Can you work these out from the drawing? Everything is in mm from the part's minimum corner. Coordinates: 2 decimals unless noted, no trailing zeros. Loops run counter-clockwise (first coordinate to the right, second up) from the corner with the lowest first, then second, coordinate; pieces in that order, holes last. Notation, with made-up numbers: M -28.75,-32.75 L 24.25,-32.75 A17 ccw 24.25,-15.75 Z; hole C -35.5,49.5 d11. An arc over 180 degrees is marked long. Use CSV: the item, a comma, the result in double quotes. Start each with the question number.
Q1. Please list where these lines run through material, in increasing order: probe 1 along X at (y, z) = (12.5, 107.95); probe 2 along Z at (x, y) = (58, 2); probe 3 along Z at (x, y) = (20.5, 3.75). Write a range as [from, to].
Q2. If we section it at A-A (z = 19.05): Please give me the cut outline in (x, y).
Q3. If we section it at D-D (x = 57.15): Please give me the cut outline in (y, z).
Q4. For pin 1 Ø18.5 at (x, z) = (38.1, 63.5) entering from -Y, with a flat end and sliding along its axis, tell me the tip position at first contact or that it passes through.
Q5. If we section it at C-C (x = 38.1): Please give me the cut outline in (y, z), and give its area (3 significant figures).
Q6. If we mould it in two halves opening along Z, with no side actions, what happens to the marked faces 1, 2 and 3? For each: +Z half, -Z half, draft (parallel to the pull), parting line (faces both ways), or undercut.
Q7. If we section it at B-B (y = 13.75): State how many separate pieces and enclosed holes the cut face has, and give its area (3 significant figures).
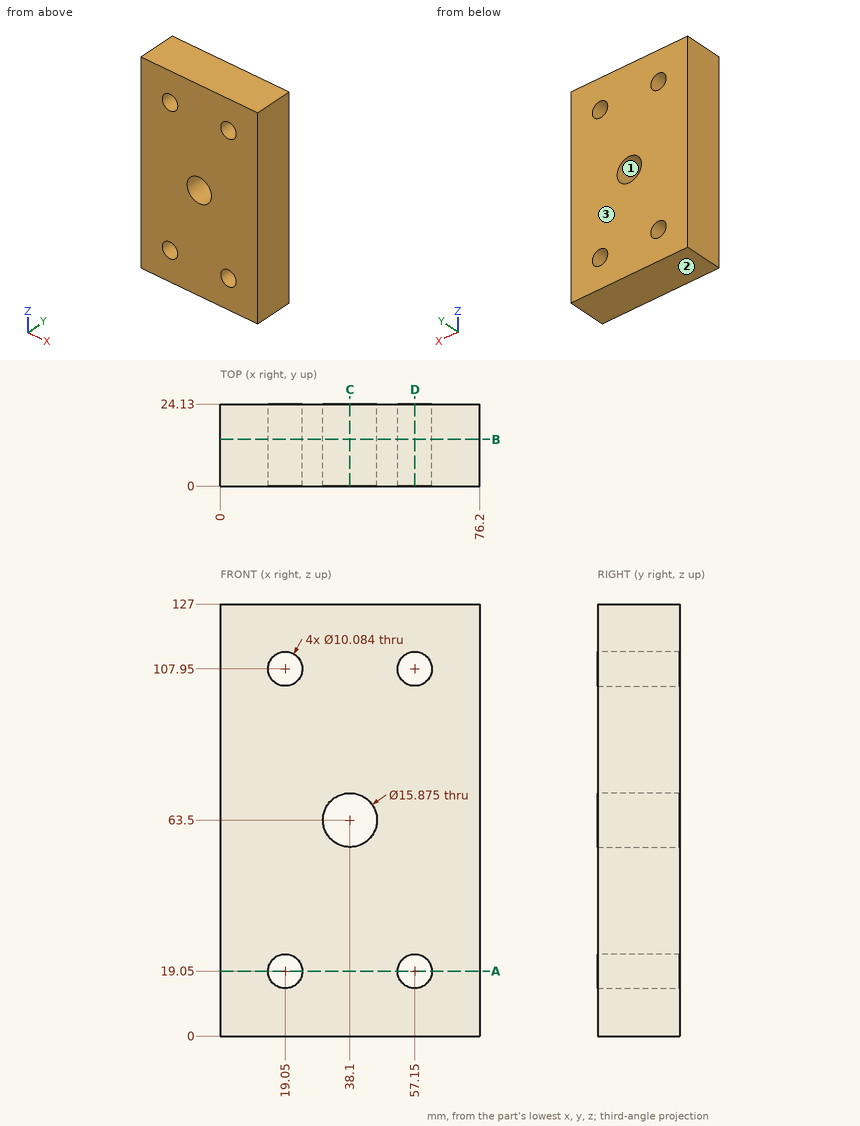
Results below:
1,probe 1,"[0, 14.01], [24.09, 52.11], [62.19, 76.2]"
1,probe 2,"[0, 14.08], [24.02, 102.98], [112.92, 127]"
1,probe 3,"[0, 14.22], [23.88, 103.12], [112.78, 127]"
2,outline,"M 0,0 L 14.01,0 L 14.01,24.13 L 0,24.13 Z; M 24.09,0 L 52.11,0 L 52.11,24.13 L 24.09,24.13 Z; M 62.19,0 L 76.2,0 L 76.2,24.13 L 62.19,24.13 Z"
3,outline,"M 0,0 L 24.13,0 L 24.13,14.01 L 0,14.01 Z; M 0,24.09 L 24.13,24.09 L 24.13,102.91 L 0,102.91 Z; M 0,112.99 L 24.13,112.99 L 24.13,127 L 0,127 Z"
4,pin 1,"y = 0"
5,outline,"M 0,0 L 24.13,0 L 24.13,55.56 L 0,55.56 Z; M 0,71.44 L 24.13,71.44 L 24.13,127 L 0,127 Z"
5,area,"2,680 mm^2"
6,face 1,"undercut"
6,face 2,"-Z half"
6,face 3,"draft"
7,separate pieces,"1"
7,enclosed holes,"5"
7,area,"9,160 mm^2"
